Geometry check sheet. Reference: drawing and pictorial views, mm from the part's lowest x, y, z. A direction names the side the tool comes from. Give positions to 0.01 mm unless a question says otherwise; leave off trailing zeros. Loops run counter-clockwise (first coordinate to the right, second up) from the corner with the lowest first, then second, coordinate; pieces in that order, holes last. Notation, with made-up numbers: (41, -16.5) -> (95, -16.5) arc R32 cw to (95, 12.5) -> close; hole circle Ø7 at (71.5, 0). An arc over 180 degrees is marked (long way). Write each question's results on one line, items separated by ' | '. Start each with the question number.
1. Cross-section at D-D on z = 13.5. Record the boundary of the cut face in (x, y), and give its area (3 significant figures).
2. Tool access check on the marked faces 4 and 5. Record the directions out of +Z, -Z, +X, -X, +Y, -Y that give a thin tool (end or side, any length) a straight path to the whole face; none if there is none.
3. Cross-section at A-A on x = 7.3. Record the boundary of the cut face in (y, z) (3 decimals).
4. Mould release check, pull along X, two halves, no side actions. Record for the marked faces 1, 2 and 3: +X half, -X half, draft (parallel to the pull), parting line (faces both ways), or undercut.
5. Cross-section at C-C on y = 6.25. Record the boundary of the cut face in (x, z) (3 decimals).
6. Material ranges on L1, parallel to Z at x = 7.3, y = 3.5 (3 decimals); L2, parallel to X at y = 8.65, z = 7.3, recorded low to high. Write a range as from..to.
7. Gauge pin test, flat ends, axial feed: pin 1 Ø1.6 at (x, y) = (13, 2.5) entering from +Z; pin 2 Ø4 at (y, z) = (6.5, 1.5) entering from -X; pin 3 Ø5 at (x, y) = (11.5, 5) entering from +Z; pin 4 Ø1 at (x, z) = (2.5, 13) entering from -Y. Record the tip position at first contact, or that the pin passes through.
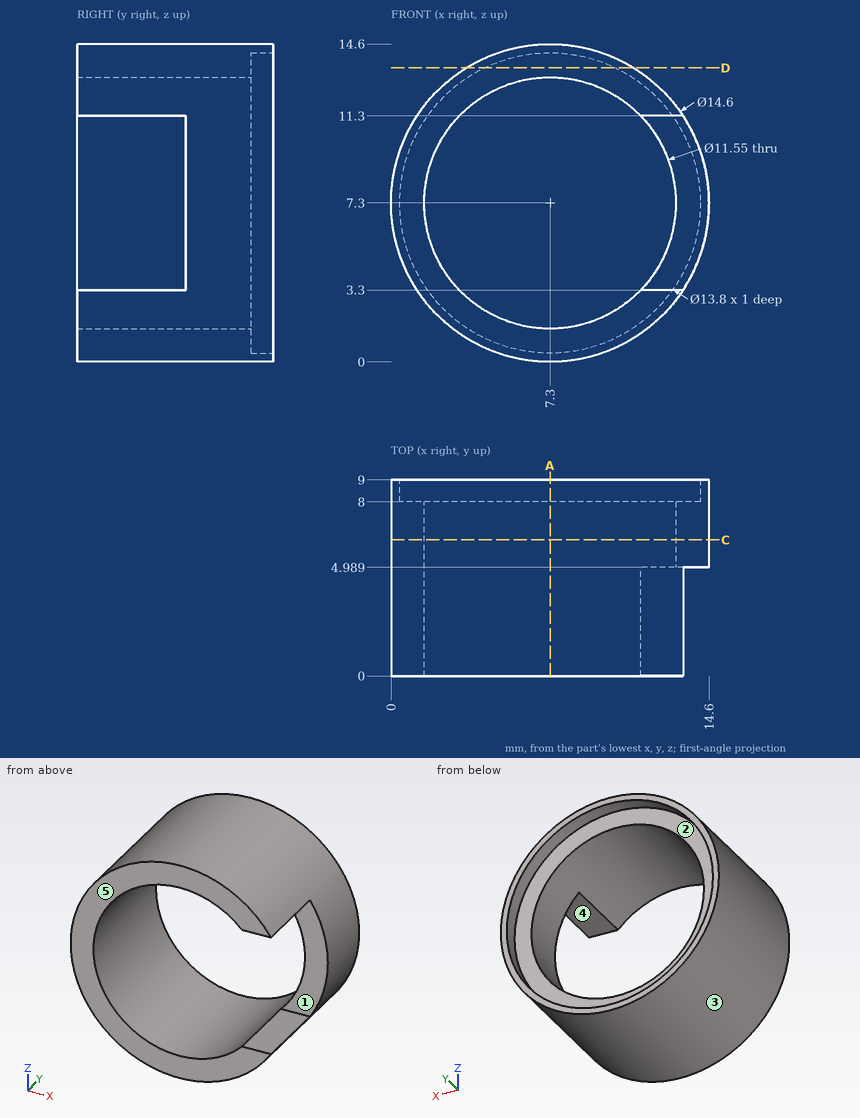
Geometry says:
1) outline: (3.45, 0) -> (11.15, 0) -> (11.15, 9) -> (10.33, 9) -> (10.33, 8) -> (4.27, 8) -> (4.27, 9) -> (3.45, 9) -> close | area: 63.3 mm^2
2) face 4: +X, -Y | face 5: +Z, -Z, +X, -X, -Y
3) outline: (0, 0) -> (9, 0) -> (9, 0.4) -> (8, 0.4) -> (8, 1.525) -> (0, 1.525) -> close; (0, 13.075) -> (8, 13.075) -> (8, 14.2) -> (9, 14.2) -> (9, 14.6) -> (0, 14.6) -> close
4) face 1: draft | face 2: undercut | face 3: parting line
5) outline: circle Ø14.6 at (7.3, 7.3); hole circle Ø11.55 at (7.3, 7.3)
6) L1: 0..1.525, 13.075..14.6 | L2: 0..0.4, 14.2..14.6
7) pin 1: z = 12.71 | pin 2: x = 1.07 | pin 3: z = 14.4 | pin 4: y = 0
